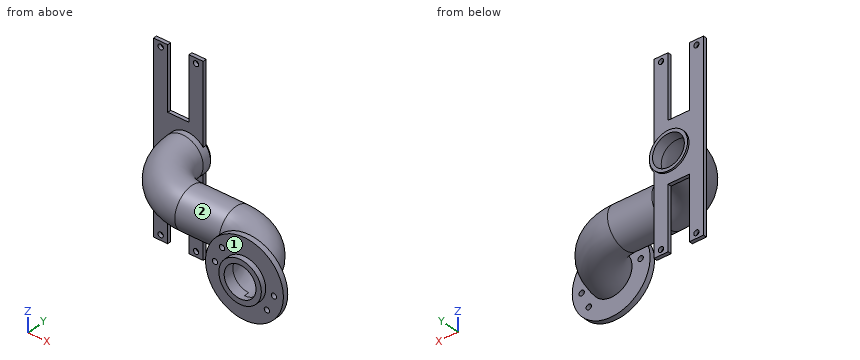
```python
from build123d import *

# Parameters (mm, degrees)
SWEEP_1_PROFILE_R   = 11.5
SWEEP_1_PROFILE_R_2 = 9
SKETCH_3_R          = 22
SKETCH_3_R_2        = 9
EXTRUDE_1_DEPTH     = 3
EXTRUDE_START       = 3
SKETCH_4_R          = 12
SKETCH_4_R_2        = 9
EXTRUDE_2_DEPTH     = 3
SKETCH_7_R          = 1.5
CUT_EXTRUDE_1_DEPTH = 10
SKETCH_8_R          = 11.5
SKETCH_8_R_2        = 9
EXTRUDE_3_DEPTH     = 5
SKETCH_9_R          = 10.8
SKETCH_9_R_2        = 9
EXTRUDE_4_DEPTH     = 1
SKETCH_10_R         = 1.5
EXTRUDE_5_DEPTH     = 2
SKETCH_11_W         = 12
SKETCH_11_H         = 36
CUT_EXTRUDE_2_DEPTH = 10


with BuildPart() as part:
    # 扫描-薄件1: sweep along a path in 草图1
    with BuildLine(Plane.XY) as sweep_1_path:
        ThreePointArc((0, 0), (-8.054563517, 19.445436483), (-27.5, 27.5))
        Line((-27.5, 27.5), (-52.5, 27.5))
        ThreePointArc((-52.5, 27.5), (-71.945436483, 35.554563517), (-80, 55))
    # 扫描-薄件1 profile (on start of the path) → 扫描-薄件1 (sweep)
    with BuildSketch(Plane(origin=(0, 0, 0), x_dir=(1, 0, 0), z_dir=(0, 1, 0))):
        Circle(SWEEP_1_PROFILE_R)
        Circle(SWEEP_1_PROFILE_R_2, mode=Mode.SUBTRACT)
    sweep(path=sweep_1_path.line)

    # 草图3 → 凸台-拉伸1 (add)
    with BuildSketch(Plane.XZ):
        Circle(SKETCH_3_R)
        Circle(SKETCH_3_R_2, mode=Mode.SUBTRACT)
    extrude(amount=-EXTRUDE_1_DEPTH)

    # 草图4 → 凸台-拉伸2 (add)
    with BuildSketch(Plane.XZ.offset(EXTRUDE_START)):
        Circle(SKETCH_4_R)
        Circle(SKETCH_4_R_2, mode=Mode.SUBTRACT)
    extrude(amount=-EXTRUDE_2_DEPTH)

    # 草图7 → 切除-拉伸1 (cut)
    with BuildSketch(Plane.XZ):
        with Locations((-12.664726672, 10.981465686)):
            Circle(SKETCH_7_R)
        with Locations((12.664726672, -10.981465686)):
            Circle(SKETCH_7_R)
        with Locations((-16.663757776, 1.818534314)):
            Circle(SKETCH_7_R)
        with Locations((16.663757776, -1.818534314)):
            Circle(SKETCH_7_R)
    extrude(amount=-CUT_EXTRUDE_1_DEPTH, mode=Mode.SUBTRACT)

    # 草图8 → 凸台-拉伸3 (add)
    with BuildSketch(Plane(origin=(0, 55, 0), x_dir=(1, 0, 0), z_dir=(0, 1, 0))):
        with Locations(Location((-80, 0, 0), (0, 0, 180))):
            Circle(SKETCH_8_R)
        with Locations(Location((-80, 0, 0), (0, 0, 180))):
            Circle(SKETCH_8_R_2, mode=Mode.SUBTRACT)
    extrude(amount=EXTRUDE_3_DEPTH)

    # 草图9 → 凸台-拉伸4 (add)
    with BuildSketch(Plane(origin=(0, 60, 0), x_dir=(1, 0, 0), z_dir=(0, 1, 0))):
        with Locations(Location((-80, 0, 0), (0, 0, 180))):
            Circle(SKETCH_9_R)
        with Locations(Location((-80, 0, 0), (0, 0, 180))):
            Circle(SKETCH_9_R_2, mode=Mode.SUBTRACT)
    extrude(amount=EXTRUDE_4_DEPTH)


with BuildPart() as body_2:
    # 草图10 → 凸台-拉伸5 (new body)
    with BuildSketch(Plane(origin=(0, 60, 0), x_dir=(1, 0, 0), z_dir=(0, 1, 0))):
        with BuildLine():
            Line((-71, 7.158910532), (-71, 53))
            Line((-71, 53), (-99, 53))
            Line((-99, 53), (-99, -53))
            Line((-99, -53), (-71, -53))
            Line((-71, -53), (-71, -7.158910532))
            ThreePointArc((-71, -7.158910532), (-91.5, 0), (-71, 7.158910532))
        make_face()
        with Locations(Location((-95, 50, 0), (0, 0, 180))):
            Circle(SKETCH_10_R, mode=Mode.SUBTRACT)
        with Locations(Location((-75, 50, 0), (0, 0, 180))):
            Circle(SKETCH_10_R, mode=Mode.SUBTRACT)
        with Locations(Location((-95, -50, 0), (0, 0, 180))):
            Circle(SKETCH_10_R, mode=Mode.SUBTRACT)
        with Locations(Location((-75, -50, 0), (0, 0, 180))):
            Circle(SKETCH_10_R, mode=Mode.SUBTRACT)
    extrude(amount=-EXTRUDE_5_DEPTH)

    # 草图11 → 切除-拉伸2 (cut)
    with BuildSketch(Plane(origin=(0, 60, 0), x_dir=(1, 0, 0), z_dir=(0, 1, 0))):
        with Locations((-85, 35)):
            Rectangle(SKETCH_11_W, SKETCH_11_H)
        with Locations((-85, -35)):
            Rectangle(SKETCH_11_W, SKETCH_11_H)
    extrude(amount=-CUT_EXTRUDE_2_DEPTH, mode=Mode.SUBTRACT)


with BuildPart() as part_1:
    add(part.part)

    # Combine 1: union body 2
    add(body_2.part)


solid = part_1.part
```
Source: CAD feature listing. Evaluate the final solid. Frame: model axes, mm. Face numbers are marked on the shaded views. A direction names the side the tool comes from. Round coordinates to 2 decimals unless told otherwise and drop trailing zeros. Write each loop counter-clockwise with the first axis right and the second up, starting at its lowest first coordinate (ties: lowest second). Pieces come first, ordered by that corner, then holes. Notation, with made-up numbers: M 11,-7.75 L 69,-7.75 A18 ccw 69,-0.75 Z; hole C 56,-20.5 d8. An arc over 180 degrees is marked long. Use CSV: the item, a comma, the result in double quotes. Start each with the question number.
Q1. Cut plane C-C on z = 34.5. Output: boundary loops of the cut face in (x, y), plus the area to 3 significant figures.
Q2. Access query for the marked faces 1 and 2. Directions: +Z, -Z, +X, -X, +Y, -Y. A direction counts if a zero-diameter tool reaches every point of the face in a straight line with its end or side. Return the directions, or none.
Q3. Cut plane A-A on z = 50. Output: boundary loops of the cut face in (x, y), plus the area to 3 significant figures.
Q4. Line query: line 1 (Z direction, x = -80, y = 59); line 2 (Z direction, x = -14.5, y = 25.5); line 3 (X direction, y = 8, z = -8). Output: solid intervals per line, ascending. Write a range as from..to.
Q5. Cut plane B-B on x = -95. Output: boundary loops of the cut face in (y, z).
Q6. Cut plane D-D on y = 56.5. Output: boundary loops of the cut face in (x, z).
Q7. First-contact query: P1, Ø4.5, axis at x = -4, z = 1, coming from the +Y side; P2, Ø8, axis at x = -21, z = -12, coming from the -Y side; P3, Ø1.6, axis at y = 59.5, z = -43, coming from the +X side; P4, Ø2.5, axis at x = -75, z = 50, coming from the +Y side. Flat tips, straight axial feed; report the tip coordinate or a pass-through.
Results found:
1,outline,"M -99,58 L -91,58 L -91,60 L -99,60 Z; M -79,58 L -71,58 L -71,60 L -79,60 Z"
1,area,"32.0 mm^2"
2,face 1,"-Y"
2,face 2,"none"
3,outline,"M -99,58 L -96.5,58 L -96.5,60 L -99,60 Z; M -93.5,58 L -91,58 L -91,60 L -93.5,60 Z; M -79,58 L -76.5,58 L -76.5,60 L -79,60 Z; M -73.5,58 L -71,58 L -71,60 L -73.5,60 Z"
3,area,"20.0 mm^2"
4,line 1,"-17..-9, 9..17"
4,line 2,"-11.45..-8.93, 8.93..11.45"
4,line 3,"-10..-5.53, 3.09..7.36"
5,outline,"M 58,-53 L 60,-53 L 60,-51.5 L 58,-51.5 Z; M 58,-48.5 L 60,-48.5 L 60,48.5 L 58,48.5 Z; M 58,51.5 L 60,51.5 L 60,53 L 58,53 Z"
6,outline,"C -80,0 d23; hole C -80,0 d18"
7,P1,"y = 32.66"
7,P2,"y = 0"
7,P3,"x = -71"
7,P4,"through"
